```python
from build123d import *

# Parameters (mm, degrees)
F1_DEPTH = 101.6
F2_R     = 50.8
F3_T     = -3.175
F4_W     = 3.175
F4_H     = 95.25
F5_DEPTH = 34.925
F7_DEPTH = 101.601
F8_R     = 12.7


with BuildPart() as f1:
    # F0 (on Front) → F1 (new body)
    with BuildSketch(Plane.XZ):
        Polygon((0, 38.1), (0, 0), (165.1, 0), (228.6, 38.1), align=None)
    extrude(amount=F1_DEPTH)

    # F2
    f2_edges = [f1.edges().sort_by_distance(p)[0] for p in [
        (165.1, -50.8, 0),
    ]]
    fillet(f2_edges, radius=F2_R)

    # F3
    f3_openings = [f1.faces().sort_by_distance(p)[0] for p in [
        (114.3, -50.8, 38.1),
    ]]
    offset(amount=F3_T, openings=f3_openings)

    # F4 (on face) → F5 (join, through all)
    with BuildSketch(Plane.XY.offset(3.175)):
        with Locations((74.6125, -50.8)):
            Rectangle(F4_W, F4_H)
        with Locations((147.6375, -50.8)):
            Rectangle(F4_W, F4_H)
    extrude(amount=F5_DEPTH)

    # F6 (on face) → F7 (cut, through all)
    with BuildSketch(Plane.XZ.offset(101.6)):
        with BuildLine():
            Line((57.15, 38.1), (19.05, 38.1))
            Line((19.05, 38.1), (19.05, 22.86))
            ThreePointArc((19.05, 22.86), (38.1, 3.81), (57.15, 22.86))
            Line((57.15, 22.86), (57.15, 38.1))
        make_face()
        with BuildLine():
            Line((133.35, 38.1), (95.25, 38.1))
            Line((95.25, 38.1), (95.25, 22.86))
            ThreePointArc((95.25, 22.86), (114.3, 3.81), (133.35, 22.86))
            Line((133.35, 22.86), (133.35, 38.1))
        make_face()
    extrude(amount=-F7_DEPTH, mode=Mode.SUBTRACT)

    # F8
    f8_edges = [f1.edges().sort_by_distance(p)[0] for p in [
        (19.05, -100.0125, 38.1),
        (57.15, -100.0125, 38.1),
        (19.05, -1.5875, 38.1),
        (57.15, -1.5875, 38.1),
        (95.25, -100.0125, 38.1),
        (133.35, -100.0125, 38.1),
        (133.35, -1.5875, 38.1),
        (95.25, -1.5875, 38.1),
    ]]
    fillet(f8_edges, radius=F8_R)


solid = f1.part
```
Input: part model. Units: mm. Frame: model coordinates. A direction names the side the tool comes from. Give positions to 0.01 mm unless a question says otherwise; leave off trailing zeros. Order: outer loops, then holes, each group sorted by start corner. A loop starts at its lowest first (then second) coordinate and runs counter-clockwise, first axis right, second up.
1. Line query: probe 1 along Y at (x, z) = (90.5, 16) (3 decimals); probe 2 along X at (y, z) = (-16.5, 29) (3 decimals); probe 3 along X at (y, z) = (-88, 17.5) (3 decimals). Output: solid intervals per line, ascending.
Computed:
probe 1: y = -101.6 to -98.425, -3.175 to 0
probe 2: x = 0 to 3.175, 73.025 to 76.2, 146.05 to 149.225, 207.262 to 213.433
probe 3: x = 0 to 3.175, 73.025 to 76.2, 146.05 to 149.225, 188.096 to 194.267
2. Cut plane A-A (x = 38.1). Return loops of the section in (y, z) (3 decimals), and give its area (3 significant figures).
Computed:
outline: (-101.6, 0) - (0, 0) - (0, 3.81) - (-3.175, 3.81) - (-3.175, 3.175) - (-98.425, 3.175) - (-98.425, 3.81) - (-101.6, 3.81) - close
area: 327 mm2
3. Pin query (flat end, axial travel): pin 1 Ø3 at (y, z) = (-100, 24) entering from -X; pin 2 Ø8 at (y, z) = (-13, 23) entering from +X; pin 3 Ø6 at (x, y) = (40, -36.5) entering from +Z (3 decimals); pin 4 Ø3 at (y, z) = (-99.5, 24.5) entering from +X. Return the tip coordinate at first contact, or that it passes through.
Computed:
pin 1: stops at x = 0
pin 2: stops at x = 210.1
pin 3: stops at z = 3.175
pin 4: stops at x = 208.43
4. Set-up query: faces 1 (the face through (111, -50, 3.175)), 2 (the face through (137.17, -99.99, 34.48)), 3 (the face through (164.4, -51.51, 1.79)). Return all of +Z, -Z, +X, -X, +Y, -Y with unobstructed straight access to the full face (end or side cutting, diameter ignored); none if empty.
Computed:
face 1: +Z
face 2: +Z, +Y, -Y
face 3: -Z, +X, +Y, -Y
5. Draft query along X for faces 4 (the face through (202.52, -50.09, 22.45)), 5 (the face through (91.43, -99.99, 34.48)), 6 (the face through (37.681, -1.61, 3.815)), 7 (the face through (113, -101.6, 2)). Return one class per face: released by +X, released by -X, zero draft, split by the parting line, or undercut.
Computed:
face 4: released by +X
face 5: undercut
face 6: undercut
face 7: zero draft
6. Cut plane B-B (y = -33). Return loops of the section in (x, z) (3 decimals).
Computed:
outline: (0, 0) - (151.029, 0) arc R50.8 ccw to (177.166, 7.239) - (228.6, 38.1) - (222.429, 38.1) - (175.532, 9.962) arc R47.625 cw to (151.029, 3.175) - (149.225, 3.175) - (149.225, 38.1) - (146.05, 38.1) - (146.05, 3.175) - (76.2, 3.175) - (76.2, 38.1) - (73.025, 38.1) - (73.025, 3.175) - (3.175, 3.175) - (3.175, 38.1) - (0, 38.1) - close
7. Cut plane C-C (x = 200). Return loops of the section in (y, z) (3 decimals), and give its area (3 significant figures).
Computed:
outline: (-101.6, 20.94) - (0, 20.94) - (0, 38.1) - (-3.175, 38.1) - (-3.175, 24.643) - (-98.425, 24.643) - (-98.425, 38.1) - (-101.6, 38.1) - close
area: 462 mm2
